Read the model definition and answer for the solid it produces. Units are mm, in the model's axes. A direction names the side the tool comes from. Round coordinates to 2 decimals unless told otherwise and drop trailing zeros. Order: outer loops, then holes, each group sorted by start corner. A loop starts at its lowest first (then second) coordinate and runs counter-clockwise, first axis right, second up. Notation, with made-up numbers: M 82.5,79.25 L 128.5,79.25 A26 cw 128.5,94.25 Z; hole C -24.5,-11 d3. An arc over 180 degrees is marked long. Answer as CSV lines item,"result".
```python
from build123d import *

# Parameters (mm, degrees)
BOSS_EXTRUDE1_DEPTH      = 5
BOSS_EXTRUDE1_DEPTH_BACK = 10
SKETCH1_R                = 15
SKETCH1_R_2              = 13
SKETCH2_R                = 15
BOSS_EXTRUDE2_DEPTH      = 2
CUT_EXTRUDE1_DEPTH       = 24.452078799
CUT_EXTRUDE1_DEPTH_BACK  = 24.452078799
SKETCH3_R                = 5.25


with BuildPart() as part:
    # Sketch1 → Boss-Extrude1 (new, two sides: drawn at the far end of the back side and taken through both)
    with BuildSketch(Plane(origin=(0, 0, 0), x_dir=(1, 0, 0), z_dir=(0, 1, 0)).offset(-BOSS_EXTRUDE1_DEPTH_BACK)):
        with Locations(Location((0, 0, 0), (0, 0, 270))):
            Circle(SKETCH1_R)
        with Locations(Location((0, 0, 0), (0, 0, 270))):
            Circle(SKETCH1_R_2, mode=Mode.SUBTRACT)
    extrude(amount=BOSS_EXTRUDE1_DEPTH + BOSS_EXTRUDE1_DEPTH_BACK)

    # Sketch2 → Boss-Extrude2 (add)
    with BuildSketch(Plane(origin=(0, 0, 0), x_dir=(1, 0, 0), z_dir=(0, 1, 0))):
        with Locations(Location((0, 0, 0), (0, 0, 270))):
            Circle(SKETCH2_R)
    extrude(amount=BOSS_EXTRUDE2_DEPTH)

    # Sketch3 → Cut-Extrude1 (cut, two sides: drawn at the far end of the back side and taken through both)
    with BuildSketch(Plane(origin=(0, 0, 0), x_dir=(1, 0, 0), z_dir=(0, 1, 0)).offset(-CUT_EXTRUDE1_DEPTH_BACK)):
        with Locations(Location((0, 0, 0), (0, 0, 270))):
            Circle(SKETCH3_R)
    extrude(amount=CUT_EXTRUDE1_DEPTH + CUT_EXTRUDE1_DEPTH_BACK, mode=Mode.SUBTRACT)


solid = part.part
```
Item 1: Determine the mould class of faces 4 (the face through (0.66, -2.605, -14.985)), 5 (the face through (13.4, 5, -0.1)), 6 (the face through (-7.91, -5.07, -10.316)) for opening direction Z: +Z half, -Z half, draft (parallel to the pull), parting line (faces both ways), or undercut.
Ans:
face 4,"parting line"
face 5,"draft"
face 6,"undercut"
Item 2: A cutting plane is placed at A-A, the plane z = 0. Determine the outline of the cut face in (x, y).
Ans:
outline,"M -15,-10 L -13,-10 L -13,0 L -5.25,0 L -5.25,2 L -13,2 L -13,5 L -15,5 Z; M 5.25,0 L 13,0 L 13,-10 L 15,-10 L 15,5 L 13,5 L 13,2 L 5.25,2 Z"
Item 3: Find the intervals of material crossed by probe 1 along X at (y, z) = (1.5, 0); probe 2 along X at (y, z) = (-7.5, 0); probe 3 along Y at (x, z) = (12.5, -2), in increasing order. Write a range as [from, to].
Ans:
probe 1,"[-15, -5.25], [5.25, 15]"
probe 2,"[-15, -13], [13, 15]"
probe 3,"[0, 2]"
Item 4: Flat-ended cylindrical pins translate along their axes: pin 1 (2 mm diameter, centred on y = 0, z = 9.5, fed in from +X); pin 2 (1.5 mm diameter, centred on y = -6, z = -4.5, fed in from +X); pin 3 (4 mm diameter, centred on y = -2, z = -8.5, fed in from -X); pin 4 (12 mm diameter, centred on x = 4.5, z = 9.5, fed in from -Y). Find the tip coordinate at first contact, or state that the pin passes through.
Ans:
pin 1,"x = 12.36"
pin 2,"x = 14.52"
pin 3,"x = -13.52"
pin 4,"y = -10"
Item 5: A cutting plane is placed at C-C, the plane y = -2.5. Determine the outline of the cut face in (x, z).
Ans:
outline,"C 0,0 d30; hole C 0,0 d26"
Item 6: A cutting plane is placed at B-B, the plane x = 0. Determine the outline of the cut face in (y, z), and give its area (3 significant figures).
Ans:
outline,"M -10,-15 L 5,-15 L 5,-13 L 2,-13 L 2,-5.25 L 0,-5.25 L 0,-13 L -10,-13 Z; M -10,13 L 0,13 L 0,5.25 L 2,5.25 L 2,13 L 5,13 L 5,15 L -10,15 Z"
area,"91.0 mm2"
Item 7: A tool of negligible diameter and unlimited length cuts with its end or side. For faces 1 (the face through (0, 0, 6)), 2 (the face through (0, 2, 6)), 3 (the face through (13.4, -10, -0.1)), from which of +Z, -Z, +X, -X, +Y, -Y can it reach the whole face along a straight path? Write none if from no direction.
Ans:
face 1,"-Y"
face 2,"+Y"
face 3,"+Z, -Z, +X, -X, -Y"
Item 8: A cutting plane is placed at D-D, the plane x = 12. Determine the outline of the cut face in (y, z), and give its area (3 significant figures).
Ans:
outline,"M -10,-9 L 5,-9 L 5,-5 L 2,-5 L 2,5 L 5,5 L 5,9 L -10,9 L -10,5 L 0,5 L 0,-5 L -10,-5 Z"
area,"140 mm2"
